Geometry check sheet. Reference: drawing and pictorial views, mm from the part's lowest x, y, z. Give positions to 0.01 mm unless a question says otherwise; leave off trailing zeros. Order: outer loops, then holes, each group sorted by start corner. A loop starts at its lowest first (then second) coordinate and runs counter-clockwise, first axis right, second up. Notation, with made-up numbers: (-1, 18) -> (58, 18) arc R22 ccw to (58, 24) -> close; hole circle Ø6 at (55, 77). An arc over 180 degrees is marked (long way). Write each question's results on one line, items separated by ' | '. Start each with the question number.
1. Cross-section at C-C, the plane z = 1.15. State how many separate pieces and enclosed holes the cut face has, then the cut area to 3 significant figures.
2. Depth check by flat-ended pin: pin 1 Ø2.5 at (x, y) = (22.5, 13.5) entering from -Z. Enter the tip coordinate at first touch or a pass-through.
3. Cross-section at A-A, the plane y = 31.5. Enter the section's corners in (x, z), then the cut area to 3 significant figures.
4. Cross-section at B-B, the plane x = 13.5. Enter the section's corners in (y, z), then the cut area to 3 significant figures.
5. Cross-section at D-D, the plane x = 22.5. Enter the section's corners in (y, z).
6. Material ranges on L1, parallel to Y at x = 13.5, z = 1.45; L2, parallel to X at y = 22.5, z = 0.7; L3, parallel to Y at x = 22, z = 2.25, recorded low to high. Write a range as from..to.
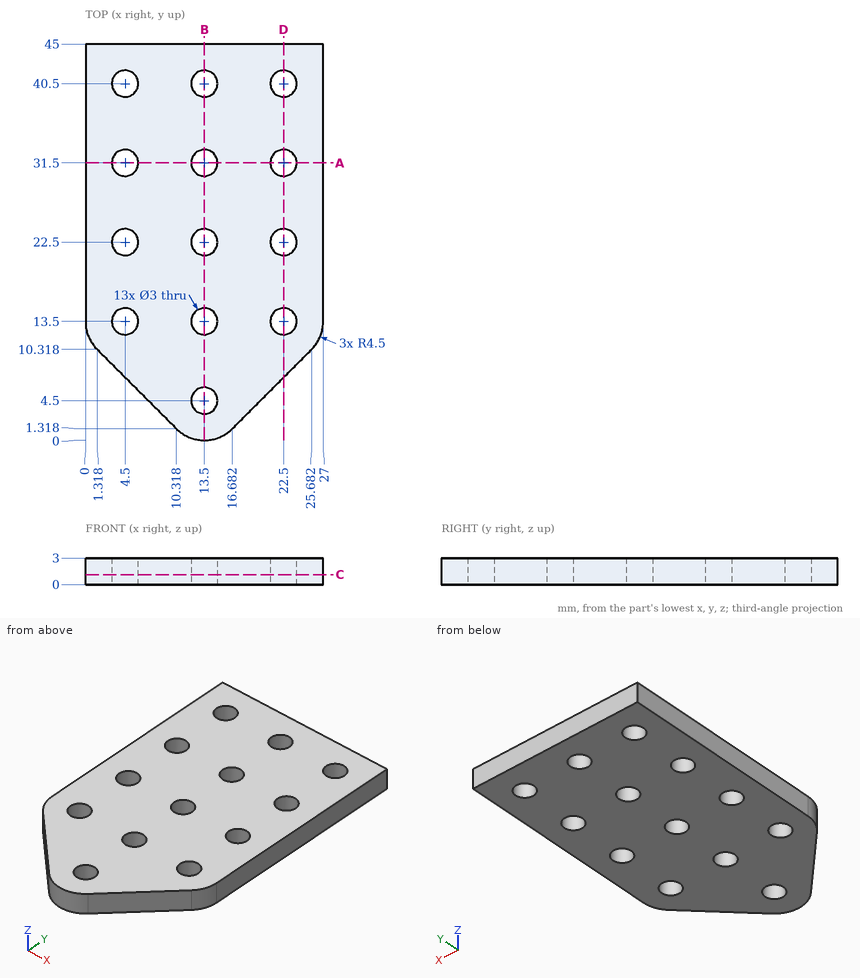
Results below:
1) separate pieces: 1 | enclosed holes: 13 | area: 986 mm²
2) pin 1: passes through
3) outline: (0, 0) -> (3, 0) -> (3, 3) -> (0, 3) -> close; (6, 0) -> (12, 0) -> (12, 3) -> (6, 3) -> close; (15, 0) -> (21, 0) -> (21, 3) -> (15, 3) -> close; (24, 0) -> (27, 0) -> (27, 3) -> (24, 3) -> close | area: 54.0 mm²
4) outline: (0, 0) -> (3, 0) -> (3, 3) -> (0, 3) -> close; (6, 0) -> (12, 0) -> (12, 3) -> (6, 3) -> close; (15, 0) -> (21, 0) -> (21, 3) -> (15, 3) -> close; (24, 0) -> (30, 0) -> (30, 3) -> (24, 3) -> close; (33, 0) -> (39, 0) -> (39, 3) -> (33, 3) -> close; (42, 0) -> (45, 0) -> (45, 3) -> (42, 3) -> close | area: 90.0 mm²
5) outline: (7.14, 0) -> (12, 0) -> (12, 3) -> (7.14, 3) -> close; (15, 0) -> (21, 0) -> (21, 3) -> (15, 3) -> close; (24, 0) -> (30, 0) -> (30, 3) -> (24, 3) -> close; (33, 0) -> (39, 0) -> (39, 3) -> (33, 3) -> close; (42, 0) -> (45, 0) -> (45, 3) -> (42, 3) -> close
6) L1: y = 0..3, 6..12, 15..21, 24..30, 33..39, 42..45 | L2: x = 0..3, 6..12, 15..21, 24..27 | L3: y = 6.64..12.09, 14.91..21.09, 23.91..30.09, 32.91..39.09, 41.91..45
